Source: CAD feature listing. Evaluate the final solid. Frame: model axes, mm. Face numbers are marked on the shaded views. A direction names the side the tool comes from. Coordinates: 2 decimals unless noted, no trailing zeros. Write each loop counter-clockwise with the first axis right and the second up, starting at its lowest first coordinate (ties: lowest second). Pieces come first, ordered by that corner, then holes. Notation, with made-up numbers: (33, 12) - (42, 12) arc R24 ccw to (42, 47) - close; hole circle Ø1 at (69, 34). An arc over 180 degrees is marked (long way). One line per question, with ' | ' between items. Start each with the question number.
Q1. Contact query for flat-ended pins moving along their axis: P1, Ø1.5, axis at x = 3, z = 0.5, coming from the +Y side; P2, Ø5, axis at y = -10.84, z = 0, coming from the +X side; P3, Ø4.5, axis at y = -10, z = -1, coming from the -X side. Output: stop coordinate, or through.
Q2. Cut plane A-A, the plane z = 0. Return loops of the section in (x, y).
Q3. Cut plane B-B, the plane y = 0.25. Return loops of the section in (x, z).
Q4. Cut plane D-D, the plane y = -10.5. Return loops of the section in (x, z).
Q5. Line query: line 1 (Y direction, x = 0.8, z = 0); line 2 (X direction, y = -8, z = -1.5); line 3 (X direction, y = -1.5, z = 2.25). Output: solid intervals per line, ascending.
Q6. Cut plane C-C, the plane x = -3.25. Return loops of the section in (y, z), plus the area to 3 significant figures.
Q7. Access query for the marked faces 1, 2 and 3. Directions: +Z, -Z, +X, -X, +Y, -Y. A direction counts if a zero-diameter tool reaches every point of the face in a straight line with its end or side. Return the directions, or none.
```python
from build123d import *

# Parameters (mm, degrees)
SKETCH1_R                 = 6
BOSS_EXTRUDE1_DEPTH       = 5
SKETCH2_W                 = 0.799850041
SKETCH2_H                 = 15.18552409
CUT_EXTRUDE1_DEPTH        = 20.213233842
F_4_0MM_DOWEL_HOLE1_D     = 4
F_4_0MM_DOWEL_HOLE1_DEPTH = 32.5
F_4_0MM_DOWEL_HOLE1_TIP   = 1.201721238


with BuildPart() as part:
    # Sketch1 → Boss-Extrude1 (new, symmetric)
    with BuildSketch(Plane.XY):
        with BuildLine():
            Line((1.5, -14.837397166), (-1.5, -14.837397166))
            Line((-1.5, -14.837397166), (-1.5, -6.837397166))
            ThreePointArc((-1.5, -6.837397166), (0, 7), (1.5, -6.837397166))
            Line((1.5, -6.837397166), (1.5, -14.837397166))
        make_face()
        Circle(SKETCH1_R, mode=Mode.SUBTRACT)
    extrude(amount=BOSS_EXTRUDE1_DEPTH, both=True)

    # Sketch2 → Cut-Extrude1 (cut, through all)
    with BuildSketch(Plane.XY.offset(5)):
        with Locations((-0.023277633, -7.592762045)):
            Rectangle(SKETCH2_W, SKETCH2_H)
    extrude(amount=-CUT_EXTRUDE1_DEPTH, mode=Mode.SUBTRACT)

    # Ø4.0mm Dowel Hole1
    with Locations(Plane.ZY.offset(1.5)):
        with Locations((0, -10.837397166)):
            Hole(F_4_0MM_DOWEL_HOLE1_D / 2, depth=F_4_0MM_DOWEL_HOLE1_DEPTH)
            with Locations((0, 0, -(F_4_0MM_DOWEL_HOLE1_DEPTH + F_4_0MM_DOWEL_HOLE1_TIP / 2))):  # 118° drill point
                Cone(0, F_4_0MM_DOWEL_HOLE1_D / 2, F_4_0MM_DOWEL_HOLE1_TIP, mode=Mode.SUBTRACT)


solid = part.part
```
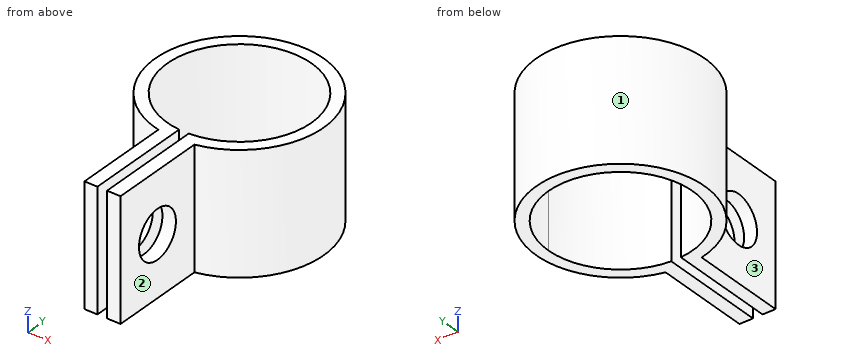
Reply:
1) P1: stops at y = 6.63 | P2: stops at x = 1.5 | P3: stops at x = -1.5
2) outline: (-1.5, -14.84) - (-0.42, -14.84) - (-0.42, -12.84) - (-1.5, -12.84) - close; (-1.5, -8.84) - (-0.42, -8.84) - (-0.42, -5.99) arc R6 cw (long way) to (0.38, -5.99) - (0.38, -8.84) - (1.5, -8.84) - (1.5, -6.84) arc R7 ccw (long way) to (-1.5, -6.84) - close; (0.38, -14.84) - (1.5, -14.84) - (1.5, -12.84) - (0.38, -12.84) - close
3) outline: (-7, -5) - (-5.99, -5) - (-5.99, 5) - (-7, 5) - close; (5.99, -5) - (7, -5) - (7, 5) - (5.99, 5) - close
4) outline: (-1.5, -5) - (-0.42, -5) - (-0.42, -1.97) - (-1.5, -1.97) - close; (-1.5, 1.97) - (-0.42, 1.97) - (-0.42, 5) - (-1.5, 5) - close; (0.38, -5) - (1.5, -5) - (1.5, -1.97) - (0.38, -1.97) - close; (0.38, 1.97) - (1.5, 1.97) - (1.5, 5) - (0.38, 5) - close
5) line 1: y = -14.84 to -12.84, -8.84 to -5.95, 5.95 to 6.95 | line 2: x = -1.5 to -0.42, 0.38 to 1.5 | line 3: x = -6.84 to -5.81, 5.81 to 6.84
6) outline: (-6.2, -5) - (-5.04, -5) - (-5.04, 5) - (-6.2, 5) - close; (5.04, -5) - (6.2, -5) - (6.2, 5) - (5.04, 5) - close | area: 23.1 mm^2
7) face 1: +Z, -Z | face 2: +Z, -Z, +X, -Y | face 3: +Z, -Z, -X, -Y
